```python
from build123d import *

# Parameters (mm, degrees)
SKETCH1_W                                            = 1510
SKETCH1_H                                            = 124.5
BOSS_EXTRUDE1_DEPTH                                  = 100
M8_TAPPED_HOLE1_D                                    = 6.8
M8_TAPPED_HOLE1_DEPTH                                = 22.25
M8_TAPPED_HOLE1_TIP                                  = 2.042926105
CBORE_FOR_M12_HEX_SOCKET_HEAD_CAP_SCREW1_D           = 13
CBORE_FOR_M12_HEX_SOCKET_HEAD_CAP_SCREW1_CBORE_D     = 20
CBORE_FOR_M12_HEX_SOCKET_HEAD_CAP_SCREW1_CBORE_DEPTH = 12.6
LPATTERN1_COUNT                                      = 18
LPATTERN1_PITCH                                      = 80


with BuildPart() as part:
    # Sketch1 → Boss-Extrude1 (new body)
    with BuildSketch(Plane.XY):
        with Locations((0, 77.25)):
            Rectangle(SKETCH1_W, SKETCH1_H)
    extrude(amount=-BOSS_EXTRUDE1_DEPTH)

    # M8 Tapped Hole1
    with Locations(Plane(origin=(0, 139.5, 0), x_dir=(1, 0, 0), z_dir=(0, 1, 0))):
        with Locations((720, 80), (720, 20), (640, 20), (640, 80), (560, 80), (560, 20), (480, 20), (480, 80), (400, 80), (400, 20), (320, 20), (320, 80), (240, 80), (240, 20), (160, 20), (160, 80), (80, 80), (80, 20), (0, 20), (0, 80), (-80, 80), (-80, 20), (-160, 20), (-160, 80), (-240, 80), (-240, 20), (-320, 20), (-320, 80), (-400, 80), (-400, 20), (-480, 20), (-480, 80), (-560, 20), (-560, 80), (-640, 20), (-640, 80), (-720, 80), (-720, 20)):
            Hole(M8_TAPPED_HOLE1_D / 2, depth=M8_TAPPED_HOLE1_DEPTH)
            with Locations((0, 0, -(M8_TAPPED_HOLE1_DEPTH + M8_TAPPED_HOLE1_TIP / 2))):  # 118° drill point
                Cone(0, M8_TAPPED_HOLE1_D / 2, M8_TAPPED_HOLE1_TIP, mode=Mode.SUBTRACT)

    # CBORE for M12 Hex Socket Head Cap Screw1 (through all)
    with Locations(Plane(origin=(0, 139.5, 0), x_dir=(1, 0, 0), z_dir=(0, 1, 0))):
        with Locations((680, 50)):
            cbore_for_m12_hex_socket_head_cap_screw1 = CounterBoreHole(CBORE_FOR_M12_HEX_SOCKET_HEAD_CAP_SCREW1_D / 2, CBORE_FOR_M12_HEX_SOCKET_HEAD_CAP_SCREW1_CBORE_D / 2, CBORE_FOR_M12_HEX_SOCKET_HEAD_CAP_SCREW1_CBORE_DEPTH)

    # LPattern1: CBORE for M12 Hex Socket Head Cap Screw1 ×18
    with Locations(*[(-i * LPATTERN1_PITCH, 0, 0) for i in range(1, LPATTERN1_COUNT)]):
        add(cbore_for_m12_hex_socket_head_cap_screw1, mode=Mode.SUBTRACT)


solid = part.part
```
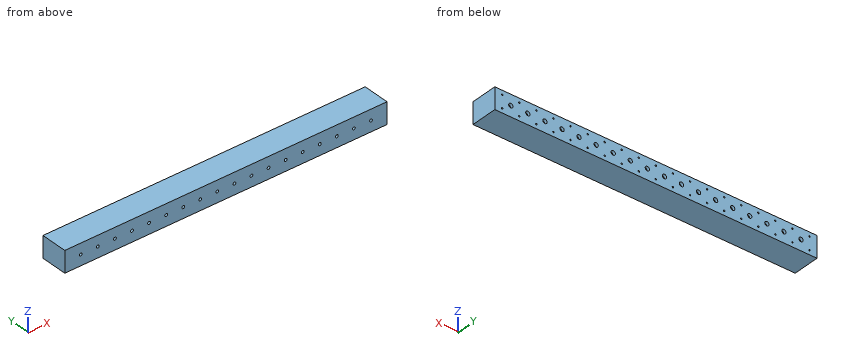
Here's how the part is built. I have some questions about the finished solid (model axes, mm). Coordinates: 2 decimals unless noted, no trailing zeros. One line per item, written item: value.
1) Suppose I cut it at A-A on y = 40. State how many separate pieces and enclosed holes the cut face has, and give its area (3 significant figures).
Model answer:
separate pieces: 1
enclosed holes: 18
area: 149,000 mm²
2) I'm going to push flat-ended pins straight in: P1, Ø16, axis at x = -680, z = -50, coming from the +Y side; P2, Ø5.5, axis at x = -640, z = -80, coming from the +Y side. Where does each tip first touch, or does it pass through?
Model answer:
P1: stops at y = 126.9
P2: stops at y = 116.86
3) I need wall thicknesses on line 1 along Z through (x, y) = (480, 134.5); line 2 along Z through (x, y) = (-520, 134); line 3 along Z through (x, y) = (-686, 93). Which ranges of each line are inside material? Lowest first, please.
Model answer:
line 1: z = -100 to -83.4, -76.6 to -23.4, -16.6 to 0
line 2: z = -100 to -60, -40 to 0
line 3: z = -100 to -52.5, -47.5 to 0
